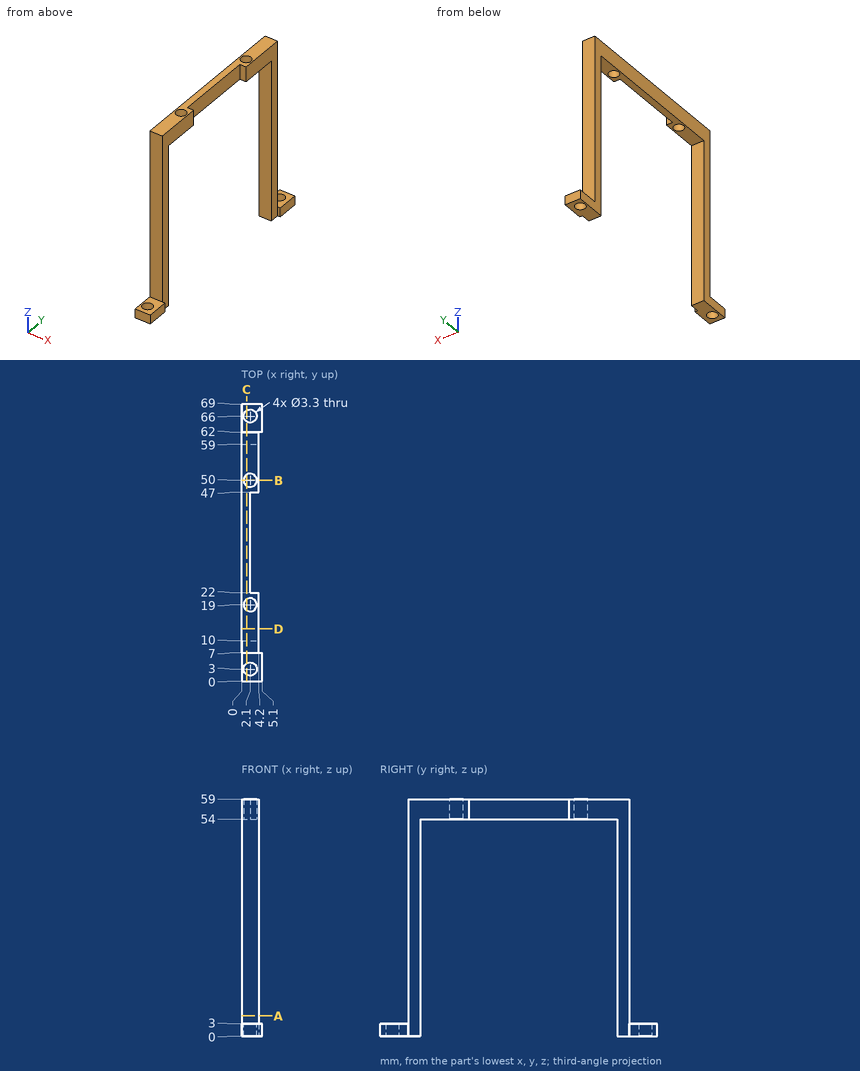
Check sheet for the drawn part. Datum: minimum x, y, z corner. Units: mm. Round coordinates to 2 decimals unless told otherwise and drop trailing zeros. Order: outer loops, then holes, each group sorted by start corner. A loop starts at its lowest first (then second) coordinate and runs counter-clockwise, first axis right, second up.
1) Section check C-C (x = 1.2). Record the boundary of the cut face in (y, z), and give its area (3 significant figures).
2) Scan lines: line 1 (Y direction, x = 2.1, z = 0.65); line 2 (X direction, y = 66, z = 1.45); line 3 (Y direction, x = 4.05, z = 18.5). Record each from-to range of solid material in increasing order.
3) Section check B-B (y = 50). Record the boundary of the cut face in (x, z).
4) Section check D-D (y = 13). Record the boundary of the cut face in (x, z).
5) Section check A-A (z = 5). Record the boundary of the cut face in (x, y), and give its area (3 significant figures).
6) Go/stop test with flat-tipped pins: pin 1 Ø2.5 at (x, y) = (3.5, 4) entering from +Z; pin 2 Ø1 at (x, z) = (3, 56) entering from +Y; pin 3 Ø3 at (x, y) = (2.1, 3) entering from +Z; pin 4 Ø7.5 at (y, z) = (13, 37) entering from +X. Record where each tip stops, or that it passes through.
Result:
1. outline: (0, 0) - (1.62, 0) - (1.62, 3) - (0, 3) - close; (4.38, 0) - (10, 0) - (10, 54) - (17.62, 54) - (17.62, 59) - (7, 59) - (7, 3) - (4.38, 3) - close; (20.38, 54) - (48.62, 54) - (48.62, 59) - (20.38, 59) - close; (51.38, 54) - (59, 54) - (59, 0) - (64.62, 0) - (64.62, 3) - (62, 3) - (62, 59) - (51.38, 59) - close; (67.38, 0) - (69, 0) - (69, 3) - (67.38, 3) - close
1. area: 597 mm2
2. line 1: y = 0 to 1.35, 4.65 to 10, 59 to 64.35, 67.65 to 69
2. line 2: x = 0 to 0.45, 3.75 to 5.1
2. line 3: y = 7 to 10, 59 to 62
3. outline: (0, 54) - (0.45, 54) - (0.45, 59) - (0, 59) - close; (3.75, 54) - (4.2, 54) - (4.2, 59) - (3.75, 59) - close
4. outline: (0, 54) - (4.2, 54) - (4.2, 59) - (0, 59) - close
5. outline: (0, 7) - (4.2, 7) - (4.2, 10) - (0, 10) - close; (0, 59) - (4.2, 59) - (4.2, 62) - (0, 62) - close
5. area: 25.2 mm2
6. pin 1: stops at z = 3
6. pin 2: stops at y = 62
6. pin 3: passes through
6. pin 4: stops at x = 4.2
